from build123d import *

# Parameters (mm, degrees)
BOSS_EXTRUDE1_DEPTH    = 1.27
SKETCH2_W              = 46.99
SKETCH2_H              = 46.99
SKETCH2_W_2            = 44.45
SKETCH2_H_2            = 44.45
BOSS_EXTRUDE2_DEPTH    = 12.7
SKETCH3_W              = 46.99
SKETCH3_H              = 46.99
BOSS_EXTRUDE3_DEPTH    = 1.27
CUT_EXTRUDE1_DEPTH     = 1.27
F_10_CLEARANCE_HOLE1_D = 4.9784
FILLET1_R              = 2.54
FILLET2_R              = 1.27
FILLET3_R              = 0.635


with BuildPart() as part:
    # Sketch1 → Boss-Extrude1 (new body)
    with BuildSketch(Plane.XY):
        Polygon((34.930491901, 50.295089045), (34.930491901, 88.395089045), (-41.269508099, 88.395089045), (-41.269508099, 12.195089045), (34.930491901, 12.195089045), align=None)
        Polygon((19.055491901, 50.295089045), (19.055491901, 72.520089045), (-25.394508099, 72.520089045), (-25.394508099, 28.070089045), (19.055491901, 28.070089045), align=None, mode=Mode.SUBTRACT)
    extrude(amount=BOSS_EXTRUDE1_DEPTH)

    # Sketch2 → Boss-Extrude2 (add)
    with BuildSketch(Plane.XY.offset(1.27)):
        with Locations((-3.169508099, 50.295089045)):
            Rectangle(SKETCH2_W, SKETCH2_H)
        with Locations((-3.169508099, 50.295089045)):
            Rectangle(SKETCH2_W_2, SKETCH2_H_2, mode=Mode.SUBTRACT)
    extrude(amount=BOSS_EXTRUDE2_DEPTH)

    # Sketch3 → Boss-Extrude3 (add)
    with BuildSketch(Plane.XY.offset(13.97)):
        with Locations((-3.169508099, 50.295089045)):
            Rectangle(SKETCH3_W, SKETCH3_H)
    extrude(amount=BOSS_EXTRUDE3_DEPTH)

    # Sketch4 → Cut-Extrude1 (cut)
    with BuildSketch(Plane.XZ.offset(-26.800089045)):
        with BuildLine():
            Line((-3.169508099, 2.54), (6.799991901, 2.54))
            ThreePointArc((6.799991901, 2.54), (7.608214952, 2.874776949), (7.942991901, 3.683))
            Line((7.942991901, 3.683), (7.942991901, 3.937))
            ThreePointArc((7.942991901, 3.937), (7.608214952, 4.745223051), (6.799991901, 5.08))
            Line((6.799991901, 5.08), (-13.139008099, 5.08))
            ThreePointArc((-13.139008099, 5.08), (-13.94723115, 4.745223051), (-14.282008099, 3.937))
            Line((-14.282008099, 3.937), (-14.282008099, 3.683))
            ThreePointArc((-14.282008099, 3.683), (-13.94723115, 2.874776949), (-13.139008099, 2.54))
            Line((-13.139008099, 2.54), (-3.169508099, 2.54))
        make_face()
    extrude(amount=-CUT_EXTRUDE1_DEPTH, mode=Mode.SUBTRACT)

    # #10 Clearance Hole1 (through all)
    with Locations(Plane(origin=(0, 0, 0), x_dir=(-1, 0, 0), z_dir=(0, 0, -1))):
        with Locations((-28.580491901, 82.181775554), (34.919508099, 82.181775554), (34.919508099, 18.681775554), (-28.580491901, 18.681775554)):
            Hole(F_10_CLEARANCE_HOLE1_D / 2)

    # Fillet1
    fillet1_edges = [part.edges().sort_by_distance(p)[0] for p in [
        (34.930491901, 12.195089045, 0.635),
        (-41.269508099, 12.195089045, 0.635),
        (-41.269508099, 88.395089045, 0.635),
        (34.930491901, 88.395089045, 0.635),
    ]]
    fillet(fillet1_edges, radius=FILLET1_R)

    # Fillet2
    fillet2_edges = [part.edges().sort_by_distance(p)[0] for p in [
        (-3.169508099, 73.790089045, 1.27),
        (20.325491901, 73.790089045, 8.255),
        (-26.664508099, 50.295089045, 1.27),
        (-26.664508099, 73.790089045, 8.255),
        (-3.169508099, 26.800089045, 1.27),
        (-26.664508099, 26.800089045, 8.255),
        (20.325491901, 50.295089045, 1.27),
        (20.325491901, 26.800089045, 8.255),
        (20.325491901, 50.295089045, 15.24),
        (-3.169508099, 73.790089045, 15.24),
        (-26.664508099, 50.295089045, 15.24),
        (-3.169508099, 26.800089045, 15.24),
    ]]
    fillet(fillet2_edges, radius=FILLET2_R - 0.0001)  # a hair under: the kernel refuses the full size

    # Fillet3
    fillet3_edges = [part.edges().sort_by_distance(p)[0] for p in [
        (19.055491901, 28.070089045, 6.985),
        (19.055491901, 72.520089045, 6.985),
        (-25.394508099, 72.520089045, 6.985),
        (-25.394508099, 28.070089045, 6.985),
        (19.055491901, 50.295089045, 13.97),
        (-3.169508099, 72.520089045, 13.97),
        (-25.394508099, 50.295089045, 13.97),
        (-3.169508099, 28.070089045, 13.97),
    ]]
    fillet(fillet3_edges, radius=FILLET3_R)


solid = part.part
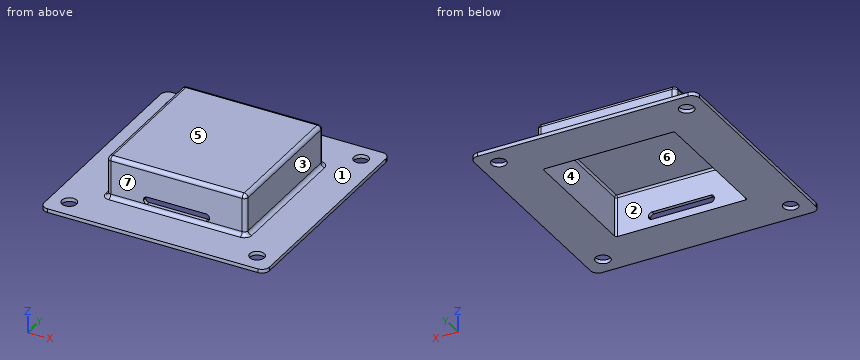
The model under review builds one solid part; all positions refer to its coordinate system, in mm. Face numbers are marked on the shaded views. A direction names the side the tool comes from. Round coordinates to 2 decimals unless told otherwise and drop trailing zeros. Order: outer loops, then holes, each group sorted by start corner. A loop starts at its lowest first (then second) coordinate and runs counter-clockwise, first axis right, second up. Notation, with made-up numbers: (40.25, 37) - (97.25, 37) arc R25 ccw to (97.25, 75) - close; hole circle Ø11 at (-21.5, 47). An arc over 180 degrees is marked (long way). Use one line per item in the form item = value.
Q1. Add section C-C on y = 31. Give the boundary of the cut face in (x, z) (1 decimal).
Response values:
outline = (-41.3, 0) - (-25.4, 0) - (-25.4, 13.3) arc R0.6 cw to (-24.8, 14) - (18.4, 14) arc R0.6 cw to (19.1, 13.3) - (19.1, 0) - (34.9, 0) - (34.9, 1.3) - (21.6, 1.3) arc R1.3 cw to (20.3, 2.5) - (20.3, 14) arc R1.3 ccw to (19.1, 15.2) - (-25.4, 15.2) arc R1.3 ccw to (-26.7, 14) - (-26.7, 2.5) arc R1.3 cw to (-27.9, 1.3) - (-41.3, 1.3) - close
Q2. Add section D-D on x = -29. Give the boundary of the cut face in (y, z), then the cut area to 3 significant figures.
Response values:
outline = (12.2, 0) - (88.4, 0) - (88.4, 1.27) - (12.2, 1.27) - close
area = 96.8 mm^2
Q3. Add section B-B on z = 7.25. Give the boundary of the cut face in (x, y) (1 decimal), then the cut area to 3 significant figures.
Response values:
outline = (-26.7, 28.1) arc R1.3 ccw to (-25.4, 26.8) - (19.1, 26.8) arc R1.3 ccw to (20.3, 28.1) - (20.3, 72.5) arc R1.3 ccw to (19.1, 73.8) - (-25.4, 73.8) arc R1.3 ccw to (-26.7, 72.5) - close; hole (-25.4, 28.7) arc R0.6 ccw to (-24.8, 28.1) - (18.4, 28.1) arc R0.6 ccw to (19.1, 28.7) - (19.1, 71.9) arc R0.6 ccw to (18.4, 72.5) - (-24.8, 72.5) arc R0.6 ccw to (-25.4, 71.9) - close
area = 231 mm^2
Q4. Clearance check with flat-ended pins moving along their axes: P1, Ø3, axis at x = -7, z = 4.5, coming from the -Y side; P2, Ø3.5, axis at y = 55.5, z = 6, coming from the +X side; P3, Ø8, axis at x = 12.5, y = 62.5, coming from the -Z side; P4, Ø4.5, axis at x = -34.92, y = 18.68, coming from the -Z side. State where each tip first meets the part, or that it passes through.
Response values:
P1 = 26.8
P2 = 20.33
P3 = 13.97
P4 = through
Q5. Mouldability with a two-part tool opening along X and no side actions: class the marked faces 1, 2, 3 and 4 as pulls with the +X half, pulls with the -X half, needs draft (parallel to the pull), parting line crosses it, or undercut.
Response values:
face_1 = needs draft
face_2 = undercut
face_3 = pulls with the +X half
face_4 = undercut
Q6. Tool access review of the marked faces 5, 6 and 7: name each direction out of +Z, -Z, +X, -X, +Y, -Y from which nothing blocks a thin tool from reaching the whole face with its end or side.
Response values:
face_5 = +Z, +X, -X, +Y, -Y
face_6 = -Z
face_7 = +Z, +X, -X, -Y
Q7. To check wall thickness, follow line 1 (Y direction, x = 11.5, z = 7.75); line 2 (X direction, y = 38, z = 2.5); line 3 (Z direction, x = -5, y = 35.5). State the ranges of each line that lie inside material, in increasing order.
Response values:
line_1 = 26.8 to 28.07, 72.52 to 73.79
line_2 = -26.67 to -25.39, 19.06 to 20.33
line_3 = 13.97 to 15.24
